Could you check a few things on this drawing? It's one solid part, dimensions in mm from its lowest x, y, z. Round coordinates to 2 decimals unless told otherwise and drop trailing zeros. Loops run counter-clockwise (first coordinate to the right, second up) from the corner with the lowest first, then second, coordinate; pieces in that order, holes last. Notation, with made-up numbers: (-15, -38.75) -> (-8, -38.75) arc R22 ccw to (-8, -3.75) -> close; hole circle Ø10 at (83.5, 38). An arc over 180 degrees is marked (long way). Use one line per item in the form item = value. Start each with the question number.
Item 1: If we section it at C-C (y = 1.1): Write out the boundary of the cut face in (x, z).
Item 2: If I drill on L1, parallel to X at y = 2.25, z = 76.2; L2, parallel to X at y = 4.15, z = 76.2; L3, parallel to Z at x = 81, y = 5.15 (1 decimal), over which ranges is the centre line in solid material (lowest first)? Write a range as [from, to].
Item 3: If we section it at A-A (z = 76.2): Write out the boundary of the cut face in (x, y).
Item 4: If we section it at B-B (x = 76.2): Write out the boundary of the cut face in (y, z).
Item 5: If we section it at D-D (x = 101.6): Write out the boundary of the cut face in (y, z).
Item 6: I'm going to push flat-ended pins straight in: pin 1 Ø1 at (y, z) = (2, 59) entering from +X; pin 2 Ø3 at (x, y) = (78, 1) entering from +Z; pin 3 Ø6.5 at (x, z) = (50.8, 76.2) entering from +Y. Where does each tip first touch, or does it pass through?
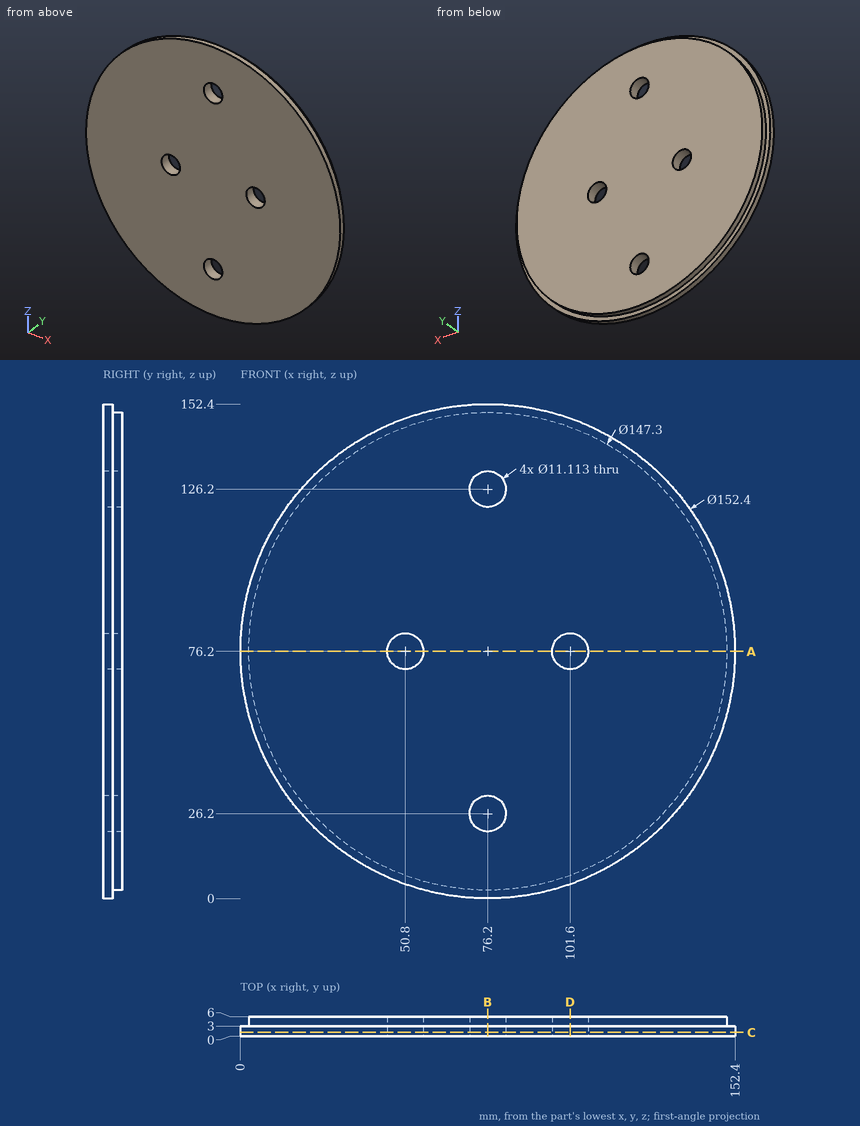
Values found:
q1.outline = circle Ø152.4 at (76.2, 76.2); hole circle Ø11.11 at (50.8, 76.2); hole circle Ø11.11 at (76.2, 26.2); hole circle Ø11.11 at (76.2, 126.2); hole circle Ø11.11 at (101.6, 76.2)
q2.L1 = [0, 45.24], [56.36, 96.04], [107.16, 152.4]
q2.L2 = [2.55, 45.24], [56.36, 96.04], [107.16, 149.85]
q2.L3 = [2.7, 23.4], [29, 123.4], [129, 149.7]
q3.outline = (0, 0) -> (45.24, 0) -> (45.24, 6) -> (2.55, 6) -> (2.55, 3) -> (0, 3) -> close; (56.36, 0) -> (96.04, 0) -> (96.04, 6) -> (56.36, 6) -> close; (107.16, 0) -> (152.4, 0) -> (152.4, 3) -> (149.85, 3) -> (149.85, 6) -> (107.16, 6) -> close
q4.outline = (0, 0) -> (3, 0) -> (3, 2.55) -> (6, 2.55) -> (6, 20.64) -> (0, 20.64) -> close; (0, 31.76) -> (6, 31.76) -> (6, 120.64) -> (0, 120.64) -> close; (0, 131.76) -> (6, 131.76) -> (6, 149.85) -> (3, 149.85) -> (3, 152.4) -> (0, 152.4) -> close
q5.outline = (0, 4.36) -> (3, 4.36) -> (3, 7.07) -> (6, 7.07) -> (6, 70.64) -> (0, 70.64) -> close; (0, 81.76) -> (6, 81.76) -> (6, 145.33) -> (3, 145.33) -> (3, 148.04) -> (0, 148.04) -> close
q6.pin_1 = 150.55
q6.pin_2 = 152.4
q6.pin_3 = through
